from build123d import *

# Parameters (mm, degrees)
CHAMFER1_SIZE      = 1.016
CUT_EXTRUDE1_DEPTH = 25.4


with BuildPart() as part:
    # Sketch1 → Revolve1 (revolve)
    with BuildSketch(Plane.XY, mode=Mode.PRIVATE) as revolve1_sk:
        with BuildLine():
            Line((9.525, 0), (0, 0))
            Line((0, 0), (0, -88.9))
            ThreePointArc((0, -88.9), (10.766948848, -82.935192091), (11.420073815, -70.64375))
            ThreePointArc((11.420073815, -70.64375), (7.585132399, -53.36790313), (11.968613609, -36.223027708))
            ThreePointArc((11.968613609, -36.223027708), (12.514442246, -34.788226477), (12.7, -33.264365659))
            Line((12.7, -33.264365659), (12.7, -25.4))
            Line((12.7, -25.4), (9.525, -25.4))
            Line((9.525, -25.4), (9.525, 0))
        make_face()
    revolve(revolve1_sk.sketch.rotate(Axis((0, 0, 0), (0, 1, 0)), 90), axis=Axis((0, 0, 0), (0, 1, 0)))

    # Chamfer1
    chamfer1_edges = [part.edges().sort_by_distance(p)[0] for p in [
        (0, 0, 9.525),
    ]]
    chamfer(chamfer1_edges, length=CHAMFER1_SIZE)

    # Sketch2 → Cut-Extrude1 (cut)
    with BuildSketch(Plane(origin=(0, 0, 0), x_dir=(-1, 0, 0), z_dir=(0, 1, 0))):
        with BuildLine():
            Line((-5.715, 7.62), (5.715, 7.62))
            ThreePointArc((5.715, 7.62), (0, 9.525), (-5.715, 7.62))
        make_face()
        with BuildLine():
            Line((-5.715, -7.62), (5.715, -7.62))
            ThreePointArc((5.715, -7.62), (0, -9.525), (-5.715, -7.62))
        make_face()
    extrude(amount=-CUT_EXTRUDE1_DEPTH, mode=Mode.SUBTRACT)


solid = part.part
Model file for the job. Use its own axes, mm. A direction names the side the tool comes from. Give positions to 0.01 mm unless a question says otherwise; leave off trailing zeros. Loops run counter-clockwise (first coordinate to the right, second up) from the corner with the lowest first, then second, coordinate; pieces in that order, holes last.
Item 1: Which spindle directions (+Z, -Z, +X, -X, +Y, -Y) get a long thin tool onto all of the face, cutting with end or side? Do faces 1 (the face through (9.524, -13.037, 0.124)), 2 (the face through (0, -13, 7.62)), 3 (the face through (-9.524, -13.037, -0.124)), 4 (the face through (0, -13, -7.62)), 5 (the face through (0, -25.4, -8)). Say none if no direction does.
Check values:
face 1: +X, +Y
face 2: +Z, +X, -X, +Y
face 3: -X, +Y
face 4: -Z, +X, -X, +Y
face 5: +Y
Item 2: Drill centre lines: line 1 along Z through (x, y) = (4.25, -7.5); line 2 along Y through (x, z) = (8.25, 6.5); line 3 along Y through (x, z) = (-9.5, 6.5). Where is each one in solid material? Low to high.
Check values:
line 1: z = -7.62 to 7.62
line 2: y = -83.34 to -68.61, -39.34 to -25.4
line 3: y = -81.57 to -70.83, -37.12 to -25.4
Item 3: Slice it at B-B (y = -60). Write the cut outline in (x, z).
Check values:
outline: circle Ø16.12 at (0, 0)
Item 4: Drop flat-ended pins along their axis: P1, Ø1.5, axis at x = -7, z = 8, coming from the +Y side; P2, Ø8, axis at x = -5.5, z = 7.5, coming from the -Y side; P3, Ø3, axis at y = -62, z = -6, coming from the +X side. Give the stop position or say it passes through.
Check values:
P1: stops at y = -25.4
P2: stops at y = -87.74
P3: stops at x = 7.21
Item 5: Slice it at A-A (y = -27). Write the cut outline in (x, z).
Check values:
outline: circle Ø25.4 at (0, 0)
